from build123d import *

# Parameters (mm, degrees)
SKETCH1_W             = 6.535180092
SKETCH1_H             = 10
SKETCH1_R             = 1.6
BOSS_EXTRUDE1_DEPTH   = 15.5
BOSS_EXTRUDE1_2_DEPTH = 15.5
BOSS_EXTRUDE1_3_DEPTH = 15.5
BOSS_EXTRUDE1_4_DEPTH = 15.5
SKETCH2_R             = 1.6
BOSS_EXTRUDE2_DEPTH   = 1
SKETCH3_W             = 2.95
SKETCH3_H             = 28.672472045
BOSS_EXTRUDE3_DEPTH   = 2.5
BOSS_EXTRUDE4_DEPTH   = 5.4
SKETCH5_W             = 2.95
SKETCH5_H             = 28.672472045
BOSS_EXTRUDE5_DEPTH   = 1
SKETCH7_W             = 109
SKETCH7_H             = 1
CUT_EXTRUDE1_DEPTH    = 9
FILLET1_R             = 3
FILLET2_R             = 3
SKETCH8_W             = 35.6
SKETCH8_H             = 2
CUT_EXTRUDE2_DEPTH    = 2


with BuildPart() as part:
    # Sketch1 → Boss-Extrude1 (new body)
    with BuildSketch(Plane(origin=(0, 0, 0), x_dir=(0, 1, 0), z_dir=(0, 0, 1))):
        with Locations((-50.739127193, -49.754164457)):
            Rectangle(SKETCH1_W, SKETCH1_H)
        with Locations(Location((-50.006717239, -49.754164457, 0), (0, 0, 270))):
            Circle(SKETCH1_R, mode=Mode.SUBTRACT)
    extrude(amount=BOSS_EXTRUDE1_DEPTH)



with BuildPart() as body_2:
    # Sketch1 → Boss-Extrude1 2 (new body)
    with BuildSketch(Plane(origin=(0, 0, 0), x_dir=(0, 1, 0), z_dir=(0, 0, 1))):
        Polygon((42.477965747, -48.576148962), (50.136732851, -40.077363358), (53.691226628, -40.077363358), (53.691226628, -48.640781304), align=None)
        with Locations(Location((49.993282761, -45.101777457, 0), (0, 0, 270))):
            Circle(SKETCH1_R, mode=Mode.SUBTRACT)
    extrude(amount=BOSS_EXTRUDE1_2_DEPTH)


with BuildPart() as body_3:
    # Sketch1 → Boss-Extrude1 3 (new body)
    with BuildSketch(Plane(origin=(0, 0, 0), x_dir=(0, 1, 0), z_dir=(0, 0, 1))):
        Polygon((53.691226628, 49.132452389), (42.477965747, 49.067820047), (50.136732851, 40.569034443), (53.691226628, 40.569034443), align=None)
        with Locations(Location((49.993282761, 45.593448542, 0), (0, 0, 90))):
            Circle(SKETCH1_R, mode=Mode.SUBTRACT)
    extrude(amount=BOSS_EXTRUDE1_3_DEPTH)


with BuildPart() as body_4:
    # Sketch1 → Boss-Extrude1 4 (new body)
    with BuildSketch(Plane(origin=(0, 0, 0), x_dir=(0, 1, 0), z_dir=(0, 0, 1))):
        with Locations((-50.739127193, 50.245835543)):
            Rectangle(SKETCH1_W, SKETCH1_H)
        with Locations(Location((-50.006717239, 50.245835543, 0), (0, 0, 90))):
            Circle(SKETCH1_R, mode=Mode.SUBTRACT)
    extrude(amount=BOSS_EXTRUDE1_4_DEPTH)


with BuildPart() as part_1:
    add(part.part)

    add(body_2.part)  # Boss-Extrude2 merges body 2

    add(body_3.part)  # Boss-Extrude2 merges body 3

    add(body_4.part)  # Boss-Extrude2 merges body 4
    # Sketch2 → Boss-Extrude2 (add)
    with BuildSketch(Plane.XY.offset(15.5)):
        Polygon((54.754164457, -47.471537147), (54.754164457, -54.006717239), (44.754164457, -54.006717239), (44.754164457, -47.471537147), (40.077363358, -47.471537147), (40.077363358, 20.986771333), (-40.569034443, 20.986771333), (-40.569034443, -47.471537147), (-45.245835543, -47.471537147), (-45.245835543, -54.006717239), (-55.245835543, -54.006717239), (-55.245835543, -47.471537147), (-55.245835543, 36.910584236), (-49.067820047, 42.477965747), (-49.132452389, 53.691226628), (-40.569034443, 53.691226628), (-40.569034443, 33.42328432), (40.077363358, 33.42328432), (40.077363358, 53.691226628), (48.640781304, 53.691226628), (48.576148962, 42.477965747), (54.754164457, 36.910584236), align=None)
        with Locations((49.754164457, -50.006717239)):
            Circle(SKETCH2_R, mode=Mode.SUBTRACT)
        with Locations((45.101777457, 49.993282761)):
            Circle(SKETCH2_R, mode=Mode.SUBTRACT)
        with Locations(Location((-45.593448542, 49.993282761, 0), (0, 0, 180))):
            Circle(SKETCH2_R, mode=Mode.SUBTRACT)
        with Locations(Location((-50.245835543, -50.006717239, 0), (0, 0, 180))):
            Circle(SKETCH2_R, mode=Mode.SUBTRACT)
    extrude(amount=BOSS_EXTRUDE2_DEPTH)

    # Sketch3 → Boss-Extrude3 (add)
    with BuildSketch(Plane.XY.offset(16.5)):
        Polygon((-52.295835543, 8.439904174), (-52.295835543, 22.986771333), (51.804164457, 22.986771333), (51.804164457, -45.813228667), (54.754164457, -45.813228667), (54.754164457, 25.986771333), (-55.245835543, 25.986771333), (-55.245835543, 8.439904174), align=None)
        with Locations((-53.770835543, -31.476992645)):
            Rectangle(SKETCH3_W, SKETCH3_H)
    extrude(amount=BOSS_EXTRUDE3_DEPTH)

    # Sketch4 → Boss-Extrude4 (add)
    with BuildSketch(Plane.XY.offset(19)):
        Polygon((-55.245835543, 25.986771333), (54.754164457, 25.986771333), (54.754164457, -45.813228667), (52.954164457, -45.813228667), (52.954164457, -43.913228667), (52.954164457, 24.086771333), (-53.445835543, 24.086771333), (-53.445835543, 8.439904174), (-55.245835543, 8.439904174), align=None)
        Polygon((-55.245835543, -45.813228667), (-53.445835543, -45.813228667), (-53.445835543, -43.913228667), (-53.445835543, -17.140756622), (-55.245835543, -17.140756622), align=None)
    extrude(amount=BOSS_EXTRUDE4_DEPTH)

    # Sketch5 → Boss-Extrude5 (add)
    with BuildSketch(Plane.XY.offset(24.4)):
        Polygon((-55.245835543, 8.439904174), (-52.295835543, 8.439904174), (-52.295835543, 22.986771333), (51.804164457, 22.986771333), (51.804164457, -45.813228667), (54.754164457, -45.813228667), (54.754164457, 25.986771333), (-55.245835543, 25.986771333), align=None)
        with Locations((-53.770835543, -31.476992645)):
            Rectangle(SKETCH5_W, SKETCH5_H)
    extrude(amount=BOSS_EXTRUDE5_DEPTH)

    # Sketch7 → Cut-Extrude1 (cut)
    with BuildSketch(Plane.XY.offset(25.4)):
        with Locations((-0.245835543, -44.313228667)):
            Rectangle(SKETCH7_W, SKETCH7_H)
    extrude(amount=-CUT_EXTRUDE1_DEPTH, mode=Mode.SUBTRACT)

    # Fillet1
    fillet1_edges = [part_1.edges().sort_by_distance(p)[0] for p in [
        (48.640781304, 53.691226628, 7.75),
        (-49.132452389, 53.691226628, 7.75),
        (-40.569034443, -47.471537147, 16),
        (-55.245835543, -54.006717239, 8.25),
        (-45.245835543, -54.006717239, 8.25),
        (40.077363358, -47.471537147, 16),
        (44.754164457, -54.006717239, 8.25),
        (54.754164457, -54.006717239, 8.25),
        (40.077363358, 53.691226628, 7.75),
        (-40.569034443, 53.691226628, 7.75),
    ]]
    fillet(fillet1_edges, radius=FILLET1_R)

    # Fillet2
    # the kernel refuses this fillet: 3 mm, written as the material it adds along each edge
    with BuildSketch(Plane(origin=(54.147639825, 37.457160078, 15.5), x_dir=(0, 0, -1), z_dir=(-0.7428654483971854, 0.6694407558385198, 0))) as fillet2_piece_1_section:
        with BuildLine():
            CenterArc((FILLET2_R, FILLET2_R), FILLET2_R, 180, 90)
            Line((0, FILLET2_R), (0, 0))
            Line((0, 0), (FILLET2_R, 0))
        make_face()
    fillet2_piece_1 = extrude(amount=26.440545017, mode=Mode.PRIVATE)
    fillet2_piece_1 = split(fillet2_piece_1, bisect_by=Plane(origin=(48.592895704, 45.383408694, 14.829727011), z_dir=(-0.9999833890252455, 0.005763824562264406, 0)), keep=Keep.TOP, mode=Mode.PRIVATE)
    fillet2_piece_1 = split(fillet2_piece_1, bisect_by=Plane(origin=(40.077363358, 45.408013282, 14.829727011), z_dir=(1, 0, 0)), keep=Keep.TOP, mode=Mode.PRIVATE)
    add(fillet2_piece_1)
    with BuildSketch(Plane(origin=(-54.63931091, 37.457160078, 15.5), x_dir=(0, 0, -1), z_dir=(0.7428654483971854, 0.6694407558385198, 0))) as fillet2_piece_2_section:
        with BuildLine():
            CenterArc((FILLET2_R, -FILLET2_R), FILLET2_R, 90, 90)
            Line((0, -FILLET2_R), (0, 0))
            Line((0, 0), (FILLET2_R, 0))
        make_face()
    fillet2_piece_2 = extrude(amount=26.440545017, mode=Mode.PRIVATE)
    fillet2_piece_2 = split(fillet2_piece_2, bisect_by=Plane(origin=(-40.569034443, 45.408013282, 14.829727011), z_dir=(-1, 0, 0)), keep=Keep.TOP, mode=Mode.PRIVATE)
    fillet2_piece_2 = split(fillet2_piece_2, bisect_by=Plane(origin=(-49.084566789, 45.383408694, 14.829727011), z_dir=(0.9999833890252455, 0.005763824562264406, 0)), keep=Keep.TOP, mode=Mode.PRIVATE)
    add(fillet2_piece_2)
    with BuildSketch(Plane(origin=(-45.245835543, -47.471537147, 15.5), x_dir=(0, 0, -1), z_dir=(-1, 0, 0)), Plane(origin=(44.754164457, -47.471537147, 15.5), x_dir=(0, 1, 0), z_dir=(1, 0, 0))) as fillet2_piece_3:
        with BuildLine():
            CenterArc((FILLET2_R, -FILLET2_R), FILLET2_R, 90, 90)
            Line((0, -FILLET2_R), (0, 0))
            Line((0, 0), (FILLET2_R, 0))
        make_face()
    extrude(amount=10)

    # Sketch8 → Cut-Extrude2 (cut)
    with BuildSketch(Plane(origin=(0, 25.986771333, 0), x_dir=(-1, 0, 0), z_dir=(0, 1, 0))):
        with Locations((0.245835543, 17.5)):
            Rectangle(SKETCH8_W, SKETCH8_H)
    extrude(amount=-CUT_EXTRUDE2_DEPTH, mode=Mode.SUBTRACT)


solid = part_1.part
Input: part model. Units: mm. Frame: model coordinates. A direction names the side the tool comes from. Round coordinates to 2 decimals unless told otherwise and drop trailing zeros. Loops run counter-clockwise (first coordinate to the right, second up) from the corner with the lowest first, then second, coordinate; pieces in that order, holes last. Notation, with made-up numbers: M 21.5,30.5 L 78.5,30.5 A13 ccw 78.5,50.5 Z; hole C 50.5,86 d2. An arc over 180 degrees is marked long. Answer as CSV lines item,"result". Start each with the question number.
(1) First-contact query: pin 1 (3 mm diameter, centred on x = 53, z = 21, fed in from -Y); pin 2 (3 mm diameter, centred on x = -47, y = -51, fed in from +Z); pin 3 (1.5 mm diameter, centred on y = -10.5, z = 14.5, fed in from +X); pin 4 (1.5 mm diameter, centred on y = -1, z = 15, fed in from -X). Flat tips, straight axial feed; report the tip coordinate or a pass-through.
(2) Section B-B, the plane y = -12.5. Output: boundary loops of the cut face in (x, z), plus the area to 3 significant figures.
(3) Section A-A, the plane z = 20.25. Output: boundary loops of the cut face in (x, y).
(4) Section C-C, the plane x = 26. Output: boundary loops of the cut face in (y, z), plus the area to 3 significant figures.
(5) Line query: line 1 (Y direction, x = 21, z = 18.25); line 2 (X direction, y = -31, z = 23); line 3 (X direction, y = -3, z = 23). Output: solid intervals per line, ascending. Write a range as [from, to].
(6) Reachability of faces 4 (the flat face through (-52.296, 16, 18)), 5 (the flat face through (-54, -44.813, 21)), 6 (the cylindrical face through (-46.148, -53.151, 8.135)), 7 (the cylindrical face through (40.933, 52.789, 8.134)) from +Z, -Z, +X, -X, +Y, -Y: full face, straight path, thin tool, end or side. Return the list, or none.
(7) Section D-D, the plane z = 6. Output: boundary loops of the cut face in (x, y).
(8) Draft query along X for faces 1 (the flat face through (-52.2, 39.655, 15.993)), 2 (the flat face through (53.4, -43.813, 20.6)), 3 (the flat face through (-54, 8.44, 21)). Return one class per face: released by +X, released by -X, zero draft, split by the parting line, or undercut.
Values found:
1,pin 1,"stops at y = -45.81"
1,pin 2,"stops at z = 16.5"
1,pin 3,"passes through"
1,pin 4,"stops at x = -55.25"
2,outline,"M -55.25,15.5 L -40.57,15.5 L -40.57,16.5 L -55.25,16.5 Z; M 40.08,15.5 L 54.75,15.5 L 54.75,25.4 L 51.8,25.4 L 51.8,24.4 L 52.95,24.4 L 52.95,19 L 51.8,19 L 51.8,16.5 L 40.08,16.5 Z"
2,area,"49.4 mm²"
3,outline,"M -55.25,-45.81 L -53.45,-45.81 L -53.45,-44.81 L -54.75,-44.81 L -54.75,-43.81 L -53.45,-43.81 L -53.45,-17.14 L -55.25,-17.14 Z; M -55.25,8.44 L -53.45,8.44 L -53.45,24.09 L 52.95,24.09 L 52.95,-43.81 L 54.25,-43.81 L 54.25,-44.81 L 52.95,-44.81 L 52.95,-45.81 L 54.75,-45.81 L 54.75,25.99 L -55.25,25.99 Z"
4,outline,"M 20.99,15.5 L 33.42,15.5 L 33.42,16.5 L 25.99,16.5 L 25.99,25.4 L 22.99,25.4 L 22.99,24.4 L 24.09,24.4 L 24.09,19 L 22.99,19 L 22.99,16.5 L 20.99,16.5 Z"
4,area,"33.2 mm²"
5,line 1,"y = [22.99, 25.99]"
5,line 2,"x = [-55.25, -53.45], [52.95, 54.75]"
5,line 3,"x = [52.95, 54.75]"
6,face 4,"+Z, -Y"
6,face 5,"+Z"
6,face 6,"+Z, -Z, -Y"
6,face 7,"+Z, -Z, +Y"
7,outline,"M -55.25,-51.01 A3 ccw -52.25,-54.01 L -48.25,-54.01 A3 ccw -45.25,-51.01 L -45.25,-47.47 L -55.25,-47.47 Z; M -49.12,50.67 L -49.07,42.48 L -40.57,50.14 L -40.57,50.69 A3 ccw -43.57,53.69 L -46.12,53.69 A3 ccw Z; M 40.08,50.14 L 48.58,42.48 L 48.62,50.67 A3 ccw 45.62,53.69 L 43.08,53.69 A3 ccw 40.08,50.69 Z; M 44.75,-51.01 A3 ccw 47.75,-54.01 L 51.75,-54.01 A3 ccw 54.75,-51.01 L 54.75,-47.47 L 44.75,-47.47 Z; hole C -50.25,-50.01 d3.2; hole C -45.59,49.99 d3.2; hole C 45.1,49.99 d3.2; hole C 49.75,-50.01 d3.2"
8,face 1,"released by -X"
8,face 2,"undercut"
8,face 3,"zero draft"
